Source: CAD feature listing. Evaluate the final solid. Frame: model axes, mm. Round coordinates to 2 decimals unless told otherwise and drop trailing zeros. Write each loop counter-clockwise with the first axis right and the second up, starting at its lowest first coordinate (ties: lowest second). Pieces come first, ordered by that corner, then holes. Notation, with made-up numbers: (58.25, -3.5) -> (89.25, -3.5) arc R10 ccw to (89.25, 10.5) -> close; hole circle Ø8 at (-38, 19.25). An arc over 180 degrees is marked (long way). Put each result on its own line as item: value.
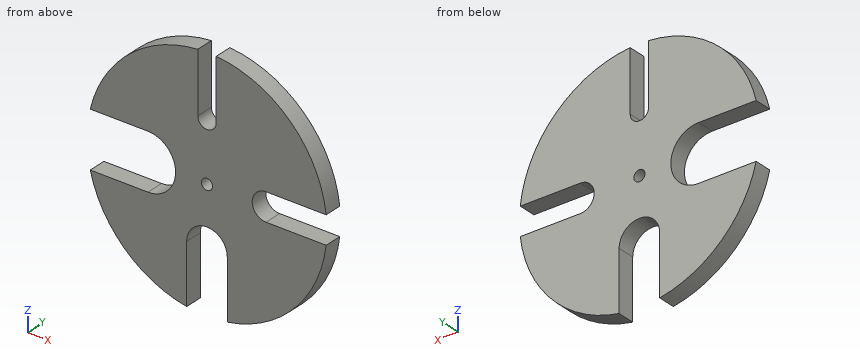
```python
from build123d import *

# Parameters (mm, degrees)
F1_DEPTH = 9.5
F3_D     = 6


with BuildPart() as f1:
    # F0 (on Front) → F1 (new body)
    with BuildSketch(Plane.XZ):
        with BuildLine():
            Line((11, -32), (11, -64.0624695122))
            ThreePointArc((11, -64.0624695122), (47.1951052283, -44.6947652695), (64.5658578507, -7.5))
            Line((64.5658578507, -7.5), (32, -7.5))
            ThreePointArc((32, -7.5), (24.5, 0), (32, 7.5))
            Line((32, 7.5), (64.5658578507, 7.5))
            ThreePointArc((64.5658578507, 7.5), (45.0653621802, 46.8413613334), (5, 64.8074069841))
            Line((5, 64.8074069841), (5, 32))
            ThreePointArc((5, 32), (0, 27), (-5, 32))
            Line((-5, 32), (-5, 64.8074069841))
            ThreePointArc((-5, 64.8074069841), (-42.2440330772, 49.4008266062), (-63.2455532034, 15))
            Line((-63.2455532034, 15), (-32, 15))
            ThreePointArc((-32, 15), (-17, 0), (-32, -15))
            Line((-32, -15), (-63.2455532034, -15))
            ThreePointArc((-63.2455532034, -15), (-44.4958652155, -47.3826759346), (-11, -64.0624695122))
            Line((-11, -64.0624695122), (-11, -32))
            ThreePointArc((-11, -32), (0, -21), (11, -32))
        make_face()
    extrude(amount=F1_DEPTH)

    # F3 (through all)
    with Locations(Plane.XZ.offset(9.5)):
        with Locations((0, 0)):
            Hole(F3_D / 2)


solid = f1.part
```
Q1. Cut plane B-B on x = 0. Output: boundary loops of the cut face in (y, z), and give its area (3 significant figures).
Ans:
outline: (-9.5, -21) -> (0, -21) -> (0, -3) -> (-9.5, -3) -> close; (-9.5, 3) -> (0, 3) -> (0, 27) -> (-9.5, 27) -> close
area: 399 mm^2
Q2. Cut plane C-C on y = -2.75. Output: boundary loops of the cut face in (x, z).
Ans:
outline: (-63.25, -15) arc R65 ccw to (-11, -64.06) -> (-11, -32) arc R11 cw to (11, -32) -> (11, -64.06) arc R65 ccw to (64.57, -7.5) -> (32, -7.5) arc R7.5 cw to (32, 7.5) -> (64.57, 7.5) arc R65 ccw to (5, 64.81) -> (5, 32) arc R5 cw to (-5, 32) -> (-5, 64.81) arc R65 ccw to (-63.25, 15) -> (-32, 15) arc R15 cw to (-32, -15) -> close; hole circle Ø6 at (0, 0)
Q3. Material intervals for line 1 (Z direction, x = 0, y = -5); line 2 (Z direction, x = -38, y = -4.5); line 3 (X direction, y = -5.25, z = 35.5), sorted ascending. Write a range as [from, to].
Ans:
line 1: z = [-21, -3], [3, 27]
line 2: z = [-52.74, -15], [15, 52.74]
line 3: x = [-54.45, -5], [5, 54.45]
Q4. Cut plane A-A on z = 0. Output: boundary loops of the cut face in (x, y).
Ans:
outline: (-17, -9.5) -> (-3, -9.5) -> (-3, 0) -> (-17, 0) -> close; (3, -9.5) -> (24.5, -9.5) -> (24.5, 0) -> (3, 0) -> close
Q5. Cut plane D-D on z = -18.5. Output: boundary loops of the cut face in (x, y), and give its area (3 significant figures).
Ans:
outline: (-62.31, -9.5) -> (62.31, -9.5) -> (62.31, 0) -> (-62.31, 0) -> close
area: 1,180 mm^2
Q6. Pin query (flat end, axial travel): pin 1 (3 mm diameter, centred on y = -4, z = -51.5, fed in from +X); pin 2 (2 mm diameter, centred on y = -3, z = -23.5, fed in from -X); pin 3 (5 mm diameter, centred on x = 41, y = -3.5, fed in from +Z); pin 4 (5 mm diameter, centred on x = -2, z = -4, fed in from +Y). Return the tip coordinate at first contact, or that it passes through.
Ans:
pin 1: stops at x = 41.53
pin 2: stops at x = -60.98
pin 3: stops at z = 52.37
pin 4: stops at y = 0
